Verification items for the finished model (mm, model axes). A direction names the side the tool comes from. Give positions to 0.01 mm unless a question says otherwise; leave off trailing zeros. Loops run counter-clockwise (first coordinate to the right, second up) from the corner with the lowest first, then second, coordinate; pieces in that order, holes last. Notation, with made-up numbers: (-3, 56) - (11, 56) arc R22 cw to (11, 76) - close; hole circle Ø8 at (19, 41). An arc over 180 degrees is marked (long way). Use one line per item in the form item = value.
```python
from build123d import *

# Parameters (mm, degrees)
SKETCH1_W           = 134
SKETCH1_H           = 63
BOSS_EXTRUDE1_DEPTH = 5
SKETCH3_R           = 12
CUT_EXTRUDE1_DEPTH  = 10
CUT_EXTRUDE2_DEPTH  = 10
BOSS_EXTRUDE2_DEPTH = 100


with BuildPart() as part:
    # Sketch1 → Boss-Extrude1 (new body)
    with BuildSketch(Plane.XY):
        Rectangle(SKETCH1_W, SKETCH1_H)
    extrude(amount=-BOSS_EXTRUDE1_DEPTH)

    # Sketch3 → Cut-Extrude1 (cut)
    with BuildSketch(Plane.XY):
        with Locations((-42, 9.071273883)):
            Circle(SKETCH3_R)
        with Locations((-14, 9.071273883)):
            Circle(SKETCH3_R)
        with Locations((14, 9.071273883)):
            Circle(SKETCH3_R)
        with Locations((42, 9.071273883)):
            Circle(SKETCH3_R)
    extrude(amount=-CUT_EXTRUDE1_DEPTH, mode=Mode.SUBTRACT)

    # Sketch4 → Cut-Extrude2 (cut)
    with BuildSketch(Plane.XY):
        Polygon((-67, -7.520628775), (-52.411804658, -7.520628775), (-45.12377265, -17.909951), (-33.648998849, -17.909951), (-29.023524966, -24.503711642), (-29.023524966, -31.5), (-67, -31.5), align=None)
        Polygon((67, -7.520628775), (67, -31.5), (29.023524966, -31.5), (29.023524966, -24.503711642), (33.648998849, -17.909951), (45.12377265, -17.909951), (52.411804658, -7.520628775), align=None)
        Polygon((-50, 31.5), (-67, 15.739047849), (-67, 31.5), align=None)
        Polygon((67, 15.739047849), (67, 31.5), (50, 31.5), align=None)
        Polygon((9.511401459, -7.520628775), (-9.511401459, -7.520628775), (-15.370004361, -13.379231677), (-8.815992906, -19.933243133), (-4.75570073, -19.933243133), (-2.290700849, -24.503711642), (0, -28.751004381), (2.290700849, -24.503711642), (4.75570073, -19.933243133), (8.815992906, -19.933243133), (15.370004361, -13.379231677), align=None)
        Polygon((-34.097223909, -10.449930226), (-29.023524966, -7.520628775), (-23.949826022, -10.449930226), (-23.949826022, -16.308533128), (-29.023524966, -19.237834579), (-34.097223909, -16.308533128), align=None)
        Polygon((29.023524966, -7.520628775), (23.949826022, -10.449930226), (23.949826022, -16.308533128), (29.023524966, -19.237834579), (34.097223909, -16.308533128), (34.097223909, -10.449930226), align=None)
    extrude(amount=-CUT_EXTRUDE2_DEPTH, mode=Mode.SUBTRACT)

    # Sketch5 → Boss-Extrude2 (add)
    with BuildSketch(Plane(origin=(50, 0, 0), x_dir=(0, 0, -1), z_dir=(1, 0, 0))):
        Polygon((-9.5, 31.5), (14.5, 31.5), (14.5, 36.149124197), (14, 36.149124197), (14, 32), (-9, 32), (-9, 36.149124197), (-9.5, 36.149124197), align=None)
    extrude(amount=-BOSS_EXTRUDE2_DEPTH)


solid = part.part
```
1. Tool access check on faces 5 (the flat face through (-67, 4, -2)), 6 (the flat face through (1, 31.5, -10)), 7 (the flat face through (39, -17.91, -2)), 8 (the flat face through (-31.525, -17.794, -2.465)). Record the directions out of +Z, -Z, +X, -X, +Y, -Y that give a thin tool (end or side, any length) a straight path to the whole face; none if there is none.
Result set:
face_5 = +Z, -Z, -X, +Y, -Y
face_6 = -Z, +X, -X, -Y
face_7 = +Z, -Z, +X, -Y
face_8 = +Z, -Z
2. Scan lines: probe 1 along Y at (x, z) = (1.5, -3); probe 2 along Y at (x, z) = (-14, -3.65); probe 3 along Z at (x, y) = (29, 19). Record each from-to range of solid material in increasing order.
Result set:
probe_1 = -31.5 to -25.97, -7.52 to 32
probe_2 = -31.5 to -14.75, -12.01 to -2.93, 21.07 to 32
probe_3 = -5 to 0
3. Section check D-D, the plane x = -14. Record the cut outline in (y, z).
Result set:
outline = (-31.5, -5) - (-14.75, -5) - (-14.75, 0) - (-31.5, 0) - close; (-12.01, -5) - (-2.93, -5) - (-2.93, 0) - (-12.01, 0) - close; (21.07, -5) - (31.5, -5) - (31.5, -14.5) - (36.15, -14.5) - (36.15, -14) - (32, -14) - (32, 9) - (36.15, 9) - (36.15, 9.5) - (31.5, 9.5) - (31.5, 0) - (21.07, 0) - close
4. Section check B-B, the plane y = -26. Record the cut outline in (x, z).
Result set:
outline = (-29.02, -5) - (-1.48, -5) - (-1.48, 0) - (-29.02, 0) - close; (1.48, -5) - (29.02, -5) - (29.02, 0) - (1.48, 0) - close
5. Section check A-A, the plane x = -42. Record the cut outline in (y, z), then the cut area to 3 significant figures.
Result set:
outline = (-17.91, -5) - (-2.93, -5) - (-2.93, 0) - (-17.91, 0) - close; (21.07, -5) - (31.5, -5) - (31.5, -14.5) - (36.15, -14.5) - (36.15, -14) - (32, -14) - (32, 9) - (36.15, 9) - (36.15, 9.5) - (31.5, 9.5) - (31.5, 0) - (21.07, 0) - close
area = 143 mm²
6. Depth check by flat-ended pin: pin 1 Ø4 at (x, z) = (-4, 2.5) entering from +Y; pin 2 Ø4 at (x, z) = (-42, 6) entering from -Y; pin 3 Ø10 at (y, z) = (20, -8.5) entering from +X. Enter the tip coordinate at first touch or a pass-through.
Result set:
pin_1 = 32
pin_2 = 31.5
pin_3 = 66.26
7. Draft check along X on faces 1 (the flat face through (58.38, 23.73, -2.46)), 2 (the flat face through (1, 34, 9.5)), 3 (the flat face through (26.45, -17.75, -2.46)), 4 (the flat face through (31.525, -17.794, -2.465)). Enter one of: released by +X, released by -X, zero draft, split by the parting line, or undercut.
Result set:
face_1 = released by +X
face_2 = zero draft
face_3 = undercut
face_4 = undercut
8. Section check C-C, the plane y = -1. Record the cut outline in (x, z).
Result set:
outline = (-67, -5) - (-48.52, -5) - (-48.52, 0) - (-67, 0) - close; (-35.48, -5) - (-20.52, -5) - (-20.52, 0) - (-35.48, 0) - close; (-7.48, -5) - (7.48, -5) - (7.48, 0) - (-7.48, 0) - close; (20.52, -5) - (35.48, -5) - (35.48, 0) - (20.52, 0) - close; (48.52, -5) - (67, -5) - (67, 0) - (48.52, 0) - close
